Verification items for this drawing (mm, ordinates from the low corner). A direction names the side the tool comes from. Round coordinates to 2 decimals unless told otherwise and drop trailing zeros. Loops run counter-clockwise (first coordinate to the right, second up) from the corner with the lowest first, then second, coordinate; pieces in that order, holes last. Notation, with made-up numbers: (81, 84) - (97, 84) arc R16 ccw to (97, 108) - close; hole circle Ø10 at (20, -1). An arc over 180 degrees is marked (long way). Use a Markdown table: item, result. Add a question column.
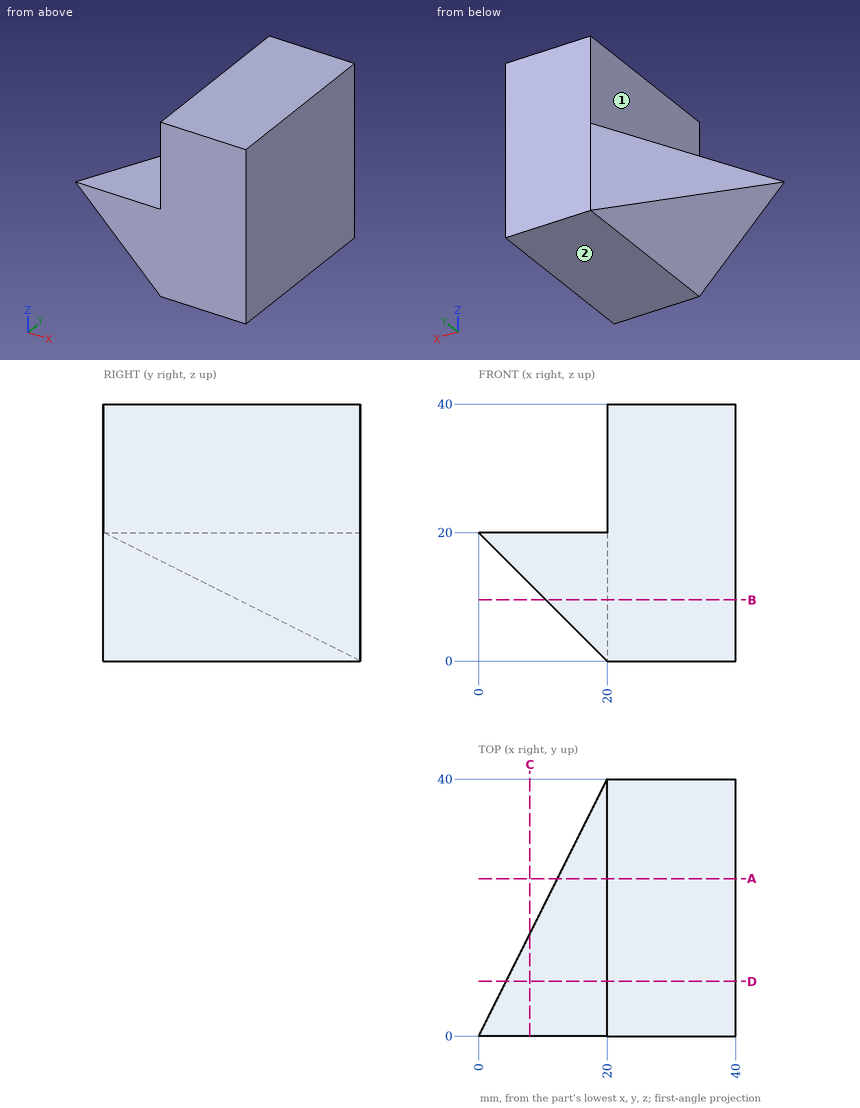
Q1. Section check C-C on x = 8. Record the cut outline in (y, z), plus the area to 3 significant figures.
Q2. Section check B-B on z = 9.5. Record the cut outline in (x, y).
Q3. Thickness scan on line 1 along X through (y, z) = (5, 28); line 2 along Y through (x, z) = (16.5, 18); line 3 along X through (y, z) = (3.5, 12). Record the ranges inside material, lowest first.
Q4. Section check D-D on y = 8.5. Record the cut outline in (x, z), plus the area to 3 significant figures.
Q5. Section check A-A on y = 24.5. Record the cut outline in (x, z).
Q6. Go/stop test with flat-tipped pins: pin 1 Ø1 at (y, z) = (16, 11.5) entering from -X; pin 2 Ø4 at (y, z) = (6, 14.5) entering from -X; pin 3 Ø6 at (x, y) = (7, 20.5) entering from +Z. Record where each tip stops, or that it passes through.
Q7. Set-up check for the marked faces 1 and 2: record each of +Z, -Z, +X, -X, +Y, -Y from which the full face is reachable in a straight line by a thin tool's end or side.
Determined:
| question | item | result |
|---|---|---|
| 1 | outline | (0, 12) - (16, 12) - (16, 20) - (0, 20) - close |
| 1 | area | 128 mm² |
| 2 | outline | (10.5, 0) - (40, 0) - (40, 40) - (20, 40) - (10.5, 21) - close |
| 3 | line 1 | x = 20 to 40 |
| 3 | line 2 | y = 0 to 33 |
| 3 | line 3 | x = 8 to 40 |
| 4 | outline | (4.25, 15.75) - (20, 0) - (40, 0) - (40, 40) - (20, 40) - (20, 20) - (4.25, 20) - close |
| 4 | area | 991 mm² |
| 5 | outline | (12.25, 7.75) - (20, 0) - (40, 0) - (40, 40) - (20, 40) - (20, 20) - (12.25, 20) - close |
| 6 | pin 1 | stops at x = 8 |
| 6 | pin 2 | stops at x = 3.5 |
| 6 | pin 3 | stops at z = 20 |
| 7 | face 1 | +Z, -X, +Y, -Y |
| 7 | face 2 | -Z, +X, -X, +Y, -Y |
